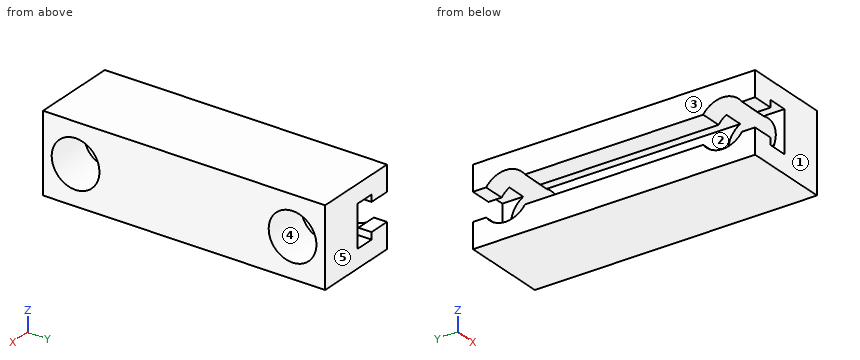
Autodesk Inventor part; units mm, degrees
ref_plane "YZ Plane" through (0, 0, 0) normal (1, 0, 0) x (0, 1, 0)
ref_plane "XZ Plane" through (0, 0, 0) normal (0, 1, 0) x (-1, 0, 0)
ref_plane "XY Plane" through (0, 0, 0) normal (0, 0, 1) x (1, 0, 0)
sketch "Sketch1" plane through (0, 0, 0) normal (0, 1, 0) x (-1, 0, 0)
  line L0 (0, 0) -> (20, 0)
  line L1 (20, 0) -> (20, 18)
  line L2 (20, 18) -> (0, 18)
  line L3 (0, 18) -> (0, 0)
  dimension "d0" = 18
  dimension "d1" = 20
extrude "Extrusion1" add sketch "Sketch1" along normal mid plane 65
sketch "Sketch2" plane through (-20, -32.5, 18) normal (-1, 0, 0) x (0, 0, 1)
  circle A0 centre (-9, 7.5) radius 3.25
  circle A1 centre (-9, 57.5) radius 3.25
  circle A2 centre (-9, 7.5) radius 5.5
  circle A3 centre (-9, 57.5) radius 5.5
  line L0 (0, 0) -> (-18, 0)
  line L1 (-18, 32.5) -> (8.866, 32.5) construction
  line L2 (-9, 65.0931) -> (-9, 0) construction
  dimension "d4" = 6.5
  dimension "d5" = 6.5
  dimension "d8" = 11
  dimension "d9" = 11
  dimension "d26" = 25
  dimension "d27" = 25
extrude "Extrusion2" cut sketch "Sketch2" against normal through all contours A0 | A1
extrude "Extrusion3" cut sketch "Sketch2" against normal blind 26
sketch "Sketch4" plane through (0, 32.5, 0) normal (0, 1, 0) x (1, 0, 0)
  line L0 (-20, 0) -> (-20, -18)
  line L1 (-20, -9) -> (2.4786, -9) construction
  line L2 (-20, -12.2) -> (-15, -12.2)
  line L3 (-15, -12.2) -> (-15, -13.8)
  line L4 (-15, -13.8) -> (-10.5, -13.8)
  line L5 (-10.5, -13.8) -> (-10.5, -4.2)
  line L6 (-10.5, -4.2) -> (-15, -4.2)
  line L7 (-15, -4.2) -> (-15, -5.8)
  line L8 (-15, -5.8) -> (-20, -5.8)
  line L9 (-20, -12.2) -> (-20, -5.8)
  point P0 (0, 0)
  dimension "d28" = 6.4
  dimension "d29" = 4.5
  dimension "d30" = 9.6
  dimension "d31" = 5
extrude "Extrusion4" cut sketch "Sketch4" against normal through all
properties part number "HeadbarHolderBracketAdjustable" material "Aluminum 6061"
The model under review builds one solid part; all positions refer to its coordinate system, in mm. Face numbers are marked on the shaded views. A direction names the side the tool comes from. Give positions to 0.01 mm unless a question says otherwise; leave off trailing zeros. Loops run counter-clockwise (first coordinate to the right, second up) from the corner with the lowest first, then second, coordinate; pieces in that order, holes last. Notation, with made-up numbers: (19.5, -30) - (26.5, -30) arc R19 cw to (26.5, 6) - close; hole circle Ø10 at (70, 65). An arc over 180 degrees is marked (long way). Answer as a JSON object with one key per item and string values.
Q1. Add section B-B on x = -18. State the section outline as (y, z) points.
Worked out:
{"outline": "(-32.5, 0) - (32.5, 0) - (32.5, 5.8) - (29.47, 5.8) arc R5.5 cw to (20.53, 5.8) - (-20.53, 5.8) arc R5.5 cw to (-29.47, 5.8) - (-32.5, 5.8) - close; (-32.5, 12.2) - (-29.47, 12.2) arc R5.5 cw to (-20.53, 12.2) - (20.53, 12.2) arc R5.5 cw to (29.47, 12.2) - (32.5, 12.2) - (32.5, 18) - (-32.5, 18) - close"}
Q2. Mouldability with a two-part tool opening along Y and no side actions: class the marked faces 3, 4 and 5 as +Y half, -Y half, draft (parallel to the pull), parting line (faces both ways), or undercut.
Worked out:
{"face 3": "draft", "face 4": "undercut", "face 5": "+Y half"}
Q3. Add section C-C on y = 25. State the section outline as (x, z) points, plus the area to 3 significant figures.
Worked out:
{"outline": "(-20, 0) - (0, 0) - (0, 3.5) - (-20, 3.5) - close; (-20, 14.5) - (0, 14.5) - (0, 18) - (-20, 18) - close", "area": "140 mm^2"}
Q4. Insertion check: pin 1 (3 mm diameter, centred on y = -10, z = 9, fed in from -X). The pin has a flat end and moves straight along its axis. Give the tip position at first contact, or say it passes through.
Worked out:
{"pin 1": "stops at x = -10.5"}
Q5. Add section D-D on x = -6.25. State the section outline as (y, z) points.
Worked out:
{"outline": "(-32.5, 0) - (32.5, 0) - (32.5, 18) - (-32.5, 18) - close; hole circle Ø11 at (-25, 9); hole circle Ø11 at (25, 9)"}
Q6. For the marked faces 1 and 2, list the 3-axis set-ups (+Z, -Z, +X, -X, +Y, -Y) from which the entire face can be reached by the end or side of a thin tool; tool diameter is ignored.
Worked out:
{"face 1": "+Z, -Z, +X, -X, -Y", "face 2": "+Y, -Y"}
Q7. Add section A-A on z = 9. State the section outline as (x, y) points.
Worked out:
{"outline": "(-10.5, -32.5) - (0, -32.5) - (0, -30.5) - (-10.5, -30.5) - close; (-10.5, -19.5) - (0, -19.5) - (0, 19.5) - (-10.5, 19.5) - close; (-10.5, 30.5) - (0, 30.5) - (0, 32.5) - (-10.5, 32.5) - close"}
Q8. To check wall thickness, follow line 1 along Y through (x, z) = (-9, 9); line 2 along X through (y, z) = (9, 13.25); line 3 along Z through (x, y) = (-18.5, 11). State the ranges of each line that lie inside material, in increasing order.
Worked out:
{"line 1": "y = -32.5 to -30.5, -19.5 to 19.5, 30.5 to 32.5", "line 2": "x = -20 to -15, -10.5 to 0", "line 3": "z = 0 to 5.8, 12.2 to 18"}
